Geometry: final body of the model. Coordinates: model frame, mm. A direction names the side the tool comes from. Round coordinates to 2 decimals unless told otherwise and drop trailing zeros. Order: outer loops, then holes, each group sorted by start corner. A loop starts at its lowest first (then second) coordinate and runs counter-clockwise, first axis right, second up. Notation, with made-up numbers: (11.5, -38) -> (18.5, -38) arc R13 ccw to (18.5, -30) -> close; hole circle Ø5 at (80.5, 55). An arc over 180 degrees is marked (long way). Put each result on its own line as item: value.
```python
from build123d import *

# Parameters (mm, degrees)
BOSS_EXTRU_2_DEPTH      = 30
ENL_V_MAT_EXTRU_1_DEPTH = 252.815317877


with BuildPart() as part:
    # Esquisse1 → Boss.-Extru.2 (new body)
    with BuildSketch(Plane.XY):
        with BuildLine():
            ThreePointArc((0, -205), (-70.078201443, -102.5), (0, 0))
            ThreePointArc((0, 0), (-4.689110868, -17.5), (0, -35))
            ThreePointArc((0, -35), (70.078201443, -137.5), (0, -240))
            ThreePointArc((0, -240), (4.689110868, -222.5), (0, -205))
        make_face()
    extrude(amount=BOSS_EXTRU_2_DEPTH)

    # Esquisse2 → Enlèv. mat.-Extru.1 (cut, through all)
    with BuildSketch(Plane.XY.offset(30)):
        Polygon((15.588457268, -111), (0, -102), (-15.588457268, -111), (-15.588457268, -129), (0, -138), (15.588457268, -129), align=None)
    extrude(amount=-ENL_V_MAT_EXTRU_1_DEPTH, mode=Mode.SUBTRACT)


solid = part.part
```
1. Cut plane C-C on x = -33. Return loops of the section in (y, z).
Ans:
outline: (-184.86, 0) -> (-20.14, 0) -> (-20.14, 30) -> (-184.86, 30) -> close
2. Cut plane A-A on z = 18. Return loops of the section in (x, y), and give its area (3 significant figures).
Ans:
outline: (0, -240) arc R110 ccw to (0, -35) arc R35 cw to (0, 0) arc R110 ccw to (0, -205) arc R35 cw to start; hole (-15.59, -129) -> (0, -138) -> (15.59, -129) -> (15.59, -111) -> (0, -102) -> (-15.59, -111) -> close
area: 19,800 mm²
3. Draft query along X for faces 1 (the face through (-7.69, -106.44, 15.21)), 2 (the face through (70.063, -135.653, 14.79)), 3 (the face through (17, -118, 30)). Return one class per face: +X half, -X half, draft (parallel to the pull), parting line (faces both ways), or undercut.
Ans:
face 1: undercut
face 2: +X half
face 3: draft
4. Cut plane D-D on y = -176.5. Return loops of the section in (x, z), and give its area (3 significant figures).
Ans:
outline: (-41.47, 0) -> (62.93, 0) -> (62.93, 30) -> (-41.47, 30) -> close
area: 3,130 mm²
5. Cut plane B-B on y = -106. Return loops of the section in (x, z).
Ans:
outline: (-70.02, 0) -> (-6.93, 0) -> (-6.93, 30) -> (-70.02, 30) -> close; (6.93, 0) -> (65.47, 0) -> (65.47, 30) -> (6.93, 30) -> close
6. Contact query for flat-ended pins moving along their axis: P1, Ø1, axis at y = -194, z = 10.5, coming from the +X side; P2, Ø8, axis at y = -69.5, z = 24, coming from the -X side; P3, Ø8, axis at x = 20, z = 23.5, coming from the -Y side. Output: stop coordinate, or through.
Ans:
P1: x = 54.76
P2: x = -66.19
P3: y = -232.22
7. Material intervals for probe 1 along Y at (x, z) = (-7.5, 16.5); probe 2 along Y at (x, z) = (6, 4); probe 3 along X at (y, z) = (-151, 21), sorted ascending.
Ans:
probe 1: -201.75 to -133.67, -106.33 to -3.25
probe 2: -237.46 to -134.54, -105.46 to -37.54
probe 3: -58.81 to 69.25
8. Set-up query: faces 4 (the face through (-4.69, -17.24, 14.79)), 5 (the face through (15.588, -120, 15)). Return all of +Z, -Z, +X, -X, +Y, -Y with unobstructed straight access to the full face (end or side cutting, diameter ignored); none if empty.
Ans:
face 4: +Z, -Z, +X
face 5: +Z, -Z
